Can you work these out from the drawing? Everything is in mm from the part's minimum corner. A direction names the side the tool comes from. Round coordinates to 2 decimals unless told otherwise and drop trailing zeros. Order: outer loops, then holes, each group sorted by start corner. A loop starts at its lowest first (then second) coordinate and runs counter-clockwise, first axis right, second up. Notation, with made-up numbers: M 38,-25 L 83,-25 A25 cw 83,-8 Z; hole C -18,-11.5 d6. An arc over 180 degrees is marked long. Write each question's results on one line, items separated by ' | '. Start each with the question number.
1. Please list where these lines run through material, in increasing order: L1, parallel to X at y = 94, z = 3.5; L2, parallel to X at y = 82, z = 24; L3, parallel to Y at x = 20.5, z = 10.75.
2. For the marked faces 1 and 2, which set-ups out of +Z, -Z, +X, -X, +Y, -Y let a thin tool reach every point of the face, with its end or its side?
3. Suppose I cut it at A-A on z = 6.75. Write out the boundary of the cut face in (x, y) (1 decimal), and give its area (3 significant figures).
4. Suppose I cut it at D-D on y = 44. Write out the boundary of the cut face in (x, z).
5. Suppose I cut it at C-C on x = 3.75. Write out the boundary of the cut face in (y, z) (1 decimal), and give its area (3 significant figures).
6. Suppose I cut it at B-B on y = 74. Write out the boundary of the cut face in (x, z) (1 decimal), and give its area (3 significant figures).
7. I'm going to push flat-ended pins straight in: pin 1 (4 mm diameter, centred on x = 22.5, y = 88, fed in from -Z) (3 decimals); pin 2 (1.5 mm diameter, centred on x = 2.5, y = 109.5, fed in from -Z); pin 3 (5.5 mm diameter, centred on x = 2, z = 16.5, fed in from +Y). Where does each tip first touch, or does it pass through?
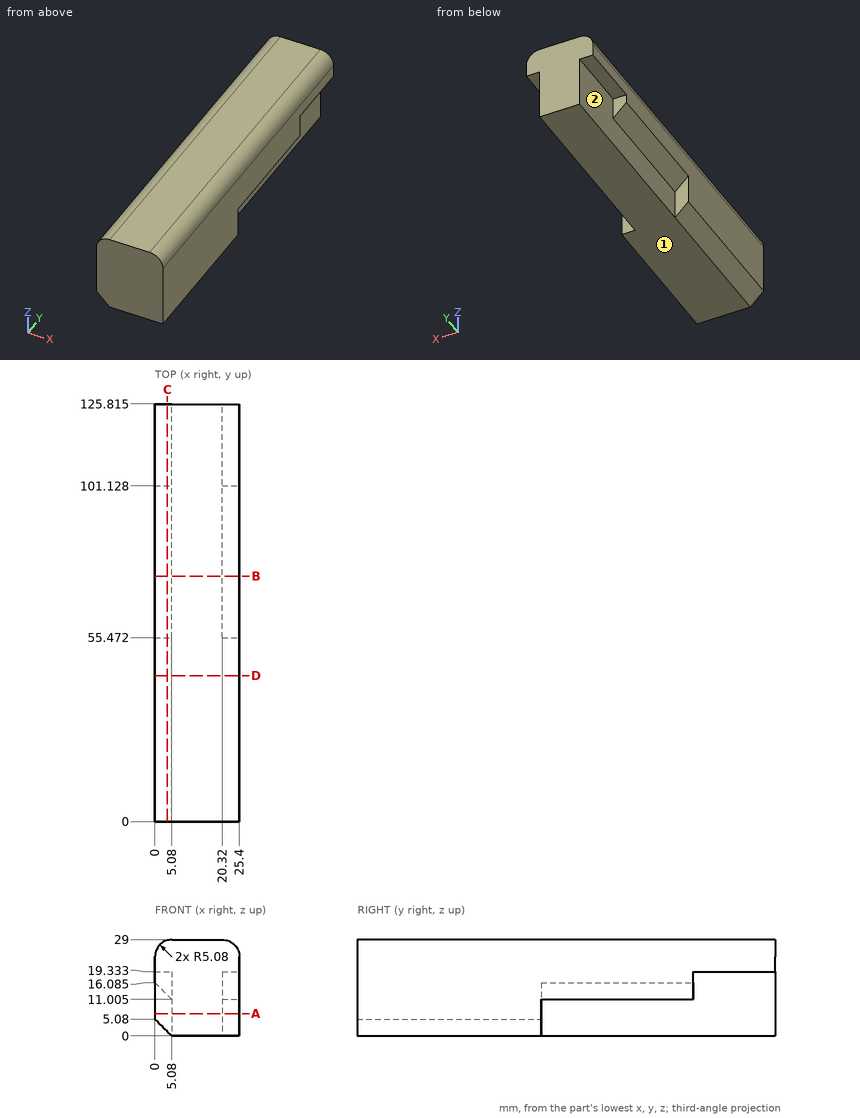
Filled sheet:
1) L1: x = 5.08 to 20.32 | L2: x = 0 to 25.4 | L3: y = 0 to 55.47
2) face 1: -Z, +X, -X, +Y, -Y | face 2: -Z, -X, +Y
3) outline: M 0,0 L 25.4,0 L 25.4,55.5 L 20.3,55.5 L 20.3,125.8 L 5.1,125.8 L 5.1,55.5 L 0,55.5 Z | area: 2,480 mm^2
4) outline: M 0,5.08 L 5.08,0 L 25.4,0 L 25.4,23.92 A5.08 ccw 20.32,29 L 5.08,29 A5.08 ccw 0,23.92 Z
5) outline: M 0,1.3 L 55.5,1.3 L 55.5,12.3 L 101.1,12.3 L 101.1,19.3 L 125.8,19.3 L 125.8,28.8 L 0,28.8 Z | area: 2,510 mm^2
6) outline: M 0,16.1 L 5.1,11 L 5.1,0 L 20.3,0 L 20.3,11 L 25.4,11 L 25.4,23.9 A5.1 ccw 20.3,29 L 5.1,29 A5.1 ccw 0,23.9 Z | area: 601 mm^2
7) pin 1: stops at z = 11.005 | pin 2: stops at z = 19.33 | pin 3: stops at y = 101.13
